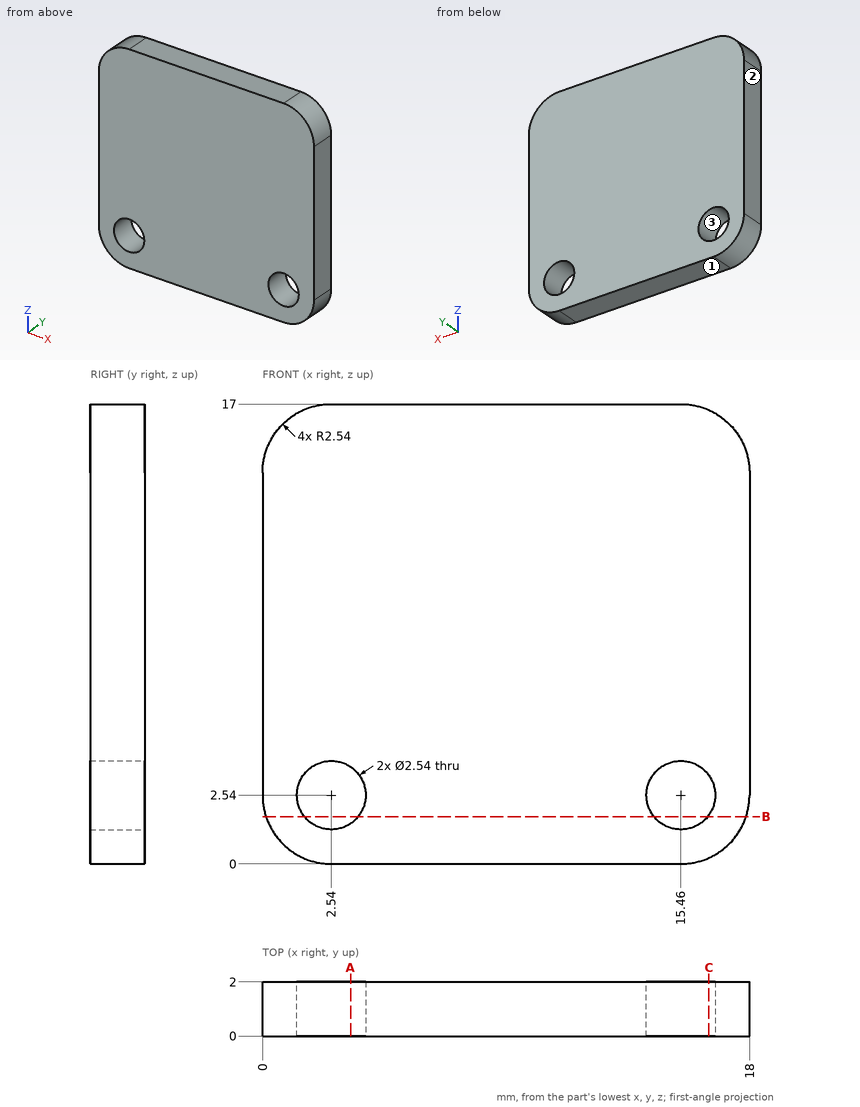
Design review of the part shown in the three views and the two pictorial views. Dimensions are in mm from the part's minimum x, y and z. Round coordinates to 2 decimals unless told otherwise and drop trailing zeros. Write each loop counter-clockwise with the first axis right and the second up, starting at its lowest first coordinate (ties: lowest second). Pieces come first, ordered by that corner, then holes. Notation, with made-up numbers: M 33.5,38.25 L 81.5,38.25 A10 ccw 81.5,44.25 Z; hole C -7.75,89.25 d5. An arc over 180 degrees is marked long. One line per item, written item: value. Start each with the question number.
1. To check wall thickness, follow probe 1 along X at (y, z) = (1.55, 2.5); probe 2 along Z at (x, y) = (15.46, 0.5); probe 3 along X at (y, z) = (1.3, 1.75). State the ranges of each line that lie inside material, in increasing order. Write a range as from..to.
2. Take a section at B-B on z = 1.75. State the section outline as (x, y) points, then the cut area to 3 significant figures.
3. Draft analysis for pull direction X (two halves, no side actions). For the marked faces 1, 2 and 3, state which applies: pulls with the +X half, pulls with the -X half, needs draft (parallel to the pull), parting line crosses it, or undercut.
4. Take a section at A-A on x = 3.25. State the section outline as (y, z) points, then the cut area to 3 significant figures.
5. Clearance check with a flat-ended pin moving along its axis: P1, Ø1.5, axis at x = 15.46, z = 2.54, coming from the +Y side. State where the tip first meets the part, or that it passes through.
6. Take a section at C-C on x = 16.5. State the section outline as (y, z) points, then the cut area to 3 significant figures.
Computed:
1. probe 1: x = 0..1.27, 3.81..14.19, 16.73..18
1. probe 2: z = 0..1.27, 3.81..17
1. probe 3: x = 0.13..1.55, 3.53..14.47, 16.45..17.87
2. outline: M 0.13,0 L 1.55,0 L 1.55,2 L 0.13,2 Z; M 3.53,0 L 14.47,0 L 14.47,2 L 3.53,2 Z; M 16.45,0 L 17.87,0 L 17.87,2 L 16.45,2 Z
2. area: 27.5 mm²
3. face 1: needs draft
3. face 2: pulls with the -X half
3. face 3: undercut
4. outline: M 0,0 L 2,0 L 2,1.49 L 0,1.49 Z; M 0,3.59 L 2,3.59 L 2,17 L 0,17 Z
4. area: 29.8 mm²
5. P1: passes through
6. outline: M 0,0.22 L 2,0.22 L 2,1.81 L 0,1.81 Z; M 0,3.27 L 2,3.27 L 2,16.78 L 0,16.78 Z
6. area: 30.2 mm²
